Answer from the drawing. Dimensions are ordinates in mm from the lowest x, y and z of the part. A direction names the side the tool comes from. Coordinates: 2 decimals unless noted, no trailing zeros. Write each loop counter-clockwise with the first axis right and the second up, starting at its lowest first coordinate (ties: lowest second). Pieces come first, ordered by that corner, then holes. Notation, with made-up numbers: (24.25, 26) -> (76.25, 26) arc R8 ccw to (76.25, 31) -> close; hole circle Ø11 at (28, 11.5). An arc over 180 degrees is marked (long way). One line per item, written item: value. Start each with the question number.
1. For the marked faces 1 and 2, determine the directions among +Z, -Z, +X, -X, +Y, -Y from which every point of the face is accessible in a straight line to the end or side of a thin tool.
2. Find section C-C, the plane z = 2. Write down the section's boundary in (x, y), and give its area (3 significant figures).
3. For a pull along X with two mould halves and no side action, classify the marked faces 3, 4 and 5 as pulls with the +X half, pulls with the -X half, needs draft (parallel to the pull), parting line crosses it, or undercut.
4. Given P1, Ø8, axis at x = 25, y = 25, coming from the +Z side; P2, Ø9.5, axis at x = 23, y = 23.5, coming from the +Z side; P3, Ø6, axis at y = 31.5, z = 3.5, coming from the +X side; P4, Ø1, axis at y = 31.5, z = 4.5, coming from the +X side, each flat-ended and moving along its own axis, determine where each tip first touches the part or whether it passes through.
5. Find section D-D, the plane x = 14.5. Write down the section's boundary in (y, z).
6. Consider line 1 along Y through (x, z) = (25, 10); line 2 along Y through (x, z) = (25, 1.45); line 3 along Z through (x, y) = (14.5, 17). Determine where each line is inside the solid, lowest interval first.
7. Find section A-A, the plane x = 25. Write down the section's boundary in (y, z), and give its area (3 significant figures).
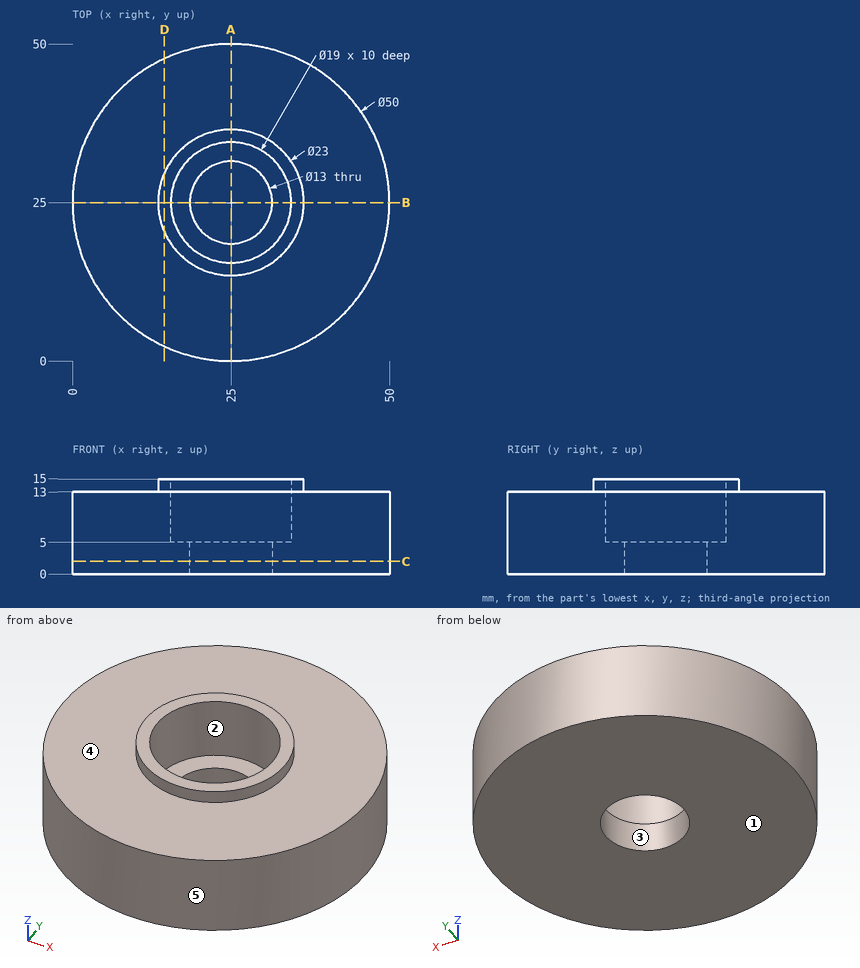
Answer block:
1. face 1: -Z, +X, -X, +Y, -Y
1. face 2: +Z
2. outline: circle Ø50 at (25, 25); hole circle Ø13 at (25, 25)
2. area: 1,830 mm2
3. face 3: undercut
3. face 4: needs draft
3. face 5: parting line crosses it
4. P1: passes through
4. P2: stops at z = 5
4. P3: stops at x = 49.75
4. P4: stops at x = 49.27
5. outline: (2.31, 0) -> (47.69, 0) -> (47.69, 13) -> (29.69, 13) -> (29.69, 15) -> (20.31, 15) -> (20.31, 13) -> (2.31, 13) -> close
6. line 1: y = 0 to 15.5, 34.5 to 50
6. line 2: y = 0 to 18.5, 31.5 to 50
6. line 3: z = 0 to 13
7. outline: (0, 0) -> (18.5, 0) -> (18.5, 5) -> (15.5, 5) -> (15.5, 15) -> (13.5, 15) -> (13.5, 13) -> (0, 13) -> close; (31.5, 0) -> (50, 0) -> (50, 13) -> (36.5, 13) -> (36.5, 15) -> (34.5, 15) -> (34.5, 5) -> (31.5, 5) -> close
7. area: 441 mm2
